Autodesk Fusion 360 part; units mm, degrees
sketch "Sketch1" plane through (0, 0, 0) normal (0, 1, 0) x (1, 0, 0)
  line L0 (0, 0) -> (10, 0)
  line L1 (10, 0) -> (10, -10)
  line L2 (0, -10) -> (0, 0)
  line L3 (10, -10) -> (9.131, -13.1109)
  arc A0 (9.131, -13.1109) -> (0, -10) centre (0, -24.956) ccw
  dimension "d1" = 10
  dimension "d2" = 10
  dimension "d3" = 3.23
extrude "Extrude1" add sketch "Sketch1" along normal blind 8
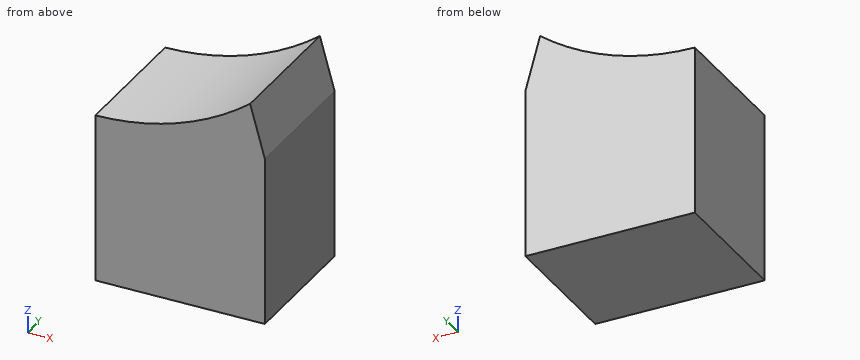
Check sheet for the modelled part. Datum: model origin and axes. Units: mm. Coordinates: 2 decimals unless noted, no trailing zeros. Loops run counter-clockwise (first coordinate to the right, second up) from the corner with the lowest first, then second, coordinate; pieces in that order, holes last. Notation, with made-up numbers: (-6, 62) -> (1, 62) arc R18 ccw to (1, 87) -> close; hole circle Ø8 at (-9.5, 44.5). An arc over 180 degrees is marked (long way). Write item = value, one per line. Start each with the question number.
1. Section check A-A on y = 4.75. Record the cut outline in (x, z).
2. Material ranges on line 1 (Z direction, x = 7.75, y = 4); line 2 (Z direction, x = 3.5, y = 2.75); line 3 (X direction, y = 5.25, z = 12), recorded low to high.
3. Section check B-B on x = 4. Record the cut outline in (y, z), then the cut area to 3 significant figures.
4. Section check C-C on x = 5.25. Record the cut outline in (y, z), then the cut area to 3 significant figures.
Responses:
q1.outline = (0, 0) -> (10, 0) -> (10, 10) -> (9.13, 13.11) arc R14.96 cw to (0, 10) -> close
q2.line_1 = 0 to 12.16
q2.line_2 = 0 to 10.42
q2.line_3 = 7.47 to 9.44
q3.outline = (0, 0) -> (8, 0) -> (8, 10.54) -> (0, 10.54) -> close
q3.area = 84.4 mm2
q4.outline = (0, 0) -> (8, 0) -> (8, 10.95) -> (0, 10.95) -> close
q4.area = 87.6 mm2
